Autodesk Fusion 360 part; units mm, degrees
sketch "Sketch1" plane through (0, 0, 0) normal (0, 0, 1) x (1, 0, 0)
  line L0 (5.7833, 3.3448) -> (5.7833, 20.3448)
  line L1 (5.7833, 20.3448) -> (35.7833, 20.3448)
  line L2 (5.7833, 3.3448) -> (55.7833, 3.3448)
  line L3 (35.7833, 20.3448) -> (5.7833, 20.3448)
  line L4 (5.7833, 20.3448) -> (5.7833, 22.8448)
  line L5 (5.7833, 22.8448) -> (35.7833, 22.8448)
  line L6 (35.7833, 22.8448) -> (35.7833, 20.3448)
  line L7 (5.7833, 3.3448) -> (55.7833, 3.3448)
  line L8 (55.7833, 3.3448) -> (55.7833, 0.8448)
  line L9 (55.7833, 0.8448) -> (5.7833, 0.8448)
  line L10 (5.7833, 0.8448) -> (5.7833, 3.3448)
  line L11 (5.7833, 22.8448) -> (3.2833, 22.8448)
  line L12 (3.2833, 22.8448) -> (3.2833, 0.8448)
  line L13 (3.2833, 0.8448) -> (5.7833, 0.8448)
  line L14 (5.7833, 0.8448) -> (5.7833, 22.8448)
  dimension "d1" = 17
  dimension "d2" = 30
  dimension "d3" = 50
  dimension "d4" = 2.5
  dimension "d5" = 2.5
  dimension "d6" = 2.5
extrude "Extrude1" add sketch "Sketch1" along normal blind 20
sketch "Sketch2" plane through (0, 0, 20) normal (0, 0, 1) x (-1, 0, 0)
  line L0 (-35.7833, -22.8448) -> (-3.2833, -22.8448)
  line L1 (-3.2833, -22.8448) -> (-3.2833, -0.8448)
  line L2 (-3.2833, -0.8448) -> (-55.7833, -0.8448)
  line L3 (-55.7833, -0.8448) -> (-55.7833, -3.3448)
  line L4 (-55.7833, -3.3448) -> (-5.7833, -3.3448)
  line L5 (-5.7833, -3.3448) -> (-5.7833, -20.3448)
  line L6 (-5.7833, -20.3448) -> (-35.7833, -20.3448)
  line L7 (-35.7833, -20.3448) -> (-35.7833, -22.8448)
sketch "Sketch3" plane through (3.2833, 0, 0) normal (-1, 0, 0) x (0, -1, 0)
  line L0 (-22.8448, 0) -> (-0.8448, 0)
  line L1 (-0.8448, 0) -> (-0.8448, 20)
  line L2 (-0.8448, 20) -> (-22.8448, 20)
  line L3 (-22.8448, 20) -> (-22.8448, 0)
  line L4 (-22.8448, 5) -> (-0.8448, 5)
  line L5 (-0.8448, 5) -> (-0.8448, 15)
  line L6 (-0.8448, 15) -> (-22.8448, 15)
  line L7 (-22.8448, 15) -> (-22.8448, 5)
  dimension "d10" = 10
extrude "Extrude2" add sketch "Sketch3" along normal blind 5 contours L1 L3 L4 L5 L6 L7
sketch "Sketch4" plane through (0, 0, 15) normal (0, 0, 1) x (-1, 0, 0)
  line L0 (-3.2833, -0.8448) -> (-3.2833, -22.8448)
  line L1 (-3.2833, -22.8448) -> (1.7167, -22.8448)
  line L2 (1.7167, -22.8448) -> (1.7167, -0.8448)
  line L3 (1.7167, -0.8448) -> (-3.2833, -0.8448)
  arc A0 (18.2167, -0.8448) -> (1.7167, -0.8448) centre (9.9667, -0.8448) ccw
  line L4 (18.2167, -0.8448) -> (23.2167, -0.8448)
  arc A1 (23.2167, -0.8448) -> (-3.2833, -0.8448) centre (9.9667, -0.8448) ccw
  dimension "d13" = 16.5
  dimension "d14" = 5
extrude "Extrude3" add sketch "Sketch4" against normal blind 10 contours L3 A0 L4 A1
fillet "Fillet1" radius 1.5 10 edges at (-20.7167, 0.8448, 15) (-20.7167, 0.8448, 5) (-18.2167, 0.8448, 10) (-23.2167, 0.8448, 10) (-9.9667, -12.4052, 5) (-9.9667, -12.4052, 15) (-9.9667, -7.4052, 5) (-1.7167, 11.8448, 5) (-9.9667, -7.4052, 15) (-1.7167, 11.8448, 15)
scale "Scale1" factor 2 about (5.7833, 20.3448, 20) bodies 1
Geometry: final body of the model. Coordinates: model frame, mm. A direction names the side the tool comes from. Round coordinates to 2 decimals unless told otherwise and drop trailing zeros. Write each loop counter-clockwise with the first axis right and the second up, starting at its lowest first coordinate (ties: lowest second). Pieces come first, ordered by that corner, then holes. Notation, with made-up numbers: M 58.5,3 L 68.5,3 A26 ccw 68.5,40 Z; hole C 25.5,24.5 d4. An arc over 180 degrees is marked long. Answer in a Markdown table with one row per item. Add a question column.
(1) Cut plane B-B, the plane z = -16. Return the cut outline in (x, y), then the cut area to 3 significant figures.
(2) Reachability of faces 1 (the face through (35, 20.345, 0)), 2 (the face through (-8.36, 3.65, 9.1)), 3 (the face through (0.783, 4, -15)), 4 (the face through (-6, -11, 10)) from +Z, -Z, +X, -X, +Y, -Y: full face, straight path, thin tool, end or side. Return the list, or none.
(3) Ray query, L1, parallel to Y at x = 47, z = -13; L2, parallel to X at y = 13, z = -6.5; L3, parallel to Y at x = 92, z = 11. Return the intervals inside material, ascending.
(4) Cut plane D-D, the plane x = 78.5. Return the cut outline in (y, z), then the cut area to 3 significant figures.
(5) Cut plane A-A, the plane x = 35. Return the cut outline in (y, z), then the cut area to 3 significant figures.
(6) Draft query along Y for faces 5 (the face through (-9.217, 4, 0)), 6 (the face through (55, -13.655, 0)), 7 (the face through (29, 25.345, 0)). Return one class per face: pulls with the +Y half, pulls with the -Y half, needs draft (parallel to the pull), parting line crosses it, or undercut.
(7) Contact query for flat-ended pins moving along their axis: pin 1 (3 mm diameter, centred on x = -47.5, z = 2.5, fed in from +Y); pin 2 (8 mm diameter, centred on x = -6.5, y = -3.5, fed in from -Z); pin 3 (4 mm diameter, centred on y = 11.5, z = -2, fed in from -X). Output: stop coordinate, or through.
(8) Cut plane C-C, the plane y = 0. Return the cut outline in (x, z).
Established:
| question | item | result |
|---|---|---|
| 1 | outline | M 0.78,-18.66 L 105.78,-18.66 L 105.78,-13.66 L 5.78,-13.66 L 5.78,20.34 L 65.78,20.34 L 65.78,25.34 L 0.78,25.34 Z |
| 1 | area | 1,020 mm² |
| 2 | face 1 | +Z, -Z, +X |
| 2 | face 2 | +Z, -X, +Y |
| 2 | face 3 | -Z, -X, +Y, -Y |
| 2 | face 4 | +Z, -X, +Y, -Y |
| 3 | L1 | -18.66 to -13.66, 20.34 to 25.34 |
| 3 | L2 | -9.22 to 5.78 |
| 3 | L3 | -18.66 to -13.66 |
| 4 | outline | M -18.66,-20 L -13.66,-20 L -13.66,20 L -18.66,20 Z |
| 4 | area | 200 mm² |
| 5 | outline | M -18.66,-20 L -13.66,-20 L -13.66,20 L -18.66,20 Z; M 20.34,-20 L 25.34,-20 L 25.34,20 L 20.34,20 Z |
| 5 | area | 400 mm² |
| 6 | face 5 | needs draft |
| 6 | face 6 | undercut |
| 6 | face 7 | pulls with the +Y half |
| 7 | pin 1 | y = -18.66 |
| 7 | pin 2 | z = -10 |
| 7 | pin 3 | x = -9.22 |
| 8 | outline | M -9.22,-7 A3 ccw -6.22,-10 L 0.78,-10 L 0.78,-20 L 5.78,-20 L 5.78,20 L 0.78,20 L 0.78,10 L -6.22,10 A3 ccw -9.22,7 Z |
